Part model, mm, in its own coordinate system. Face numbers are marked on the shaded views. A direction names the side the tool comes from. Give positions to 0.01 mm unless a question says otherwise; leave off trailing zeros. Order: outer loops, then holes, each group sorted by start corner. A loop starts at its lowest first (then second) coordinate and runs counter-clockwise, first axis right, second up. Notation, with made-up numbers: M 21.5,75 L 56.5,75 A16 cw 56.5,80 Z; hole C 38,31.25 d4. An arc over 180 degrees is marked long. Return JSON: item names as keys, results as strings.
from build123d import *

# Parameters (mm, degrees)
SKETCH1_R     = 6.55
BODY_DEPTH    = 7.3
FLOOR_2_DEPTH = 2.2


with BuildPart() as part:
    # Sketch1 → Body (new body)
    with BuildSketch(Plane(origin=(0, 0, 0), x_dir=(1, 0, 0), z_dir=(0, 1, 0))):
        with BuildLine():
            Line((3, -8.006403687), (15.495614035, -3.324296268))
            ThreePointArc((15.495614035, -3.324296268), (17.8, 0), (15.495614035, 3.324296268))
            Line((15.495614035, 3.324296268), (3, 8.006403687))
            ThreePointArc((3, 8.006403687), (-0.436058681, 8.538873042), (-3.8, 7.659144861))
            Line((-3.8, 7.659144861), (-8.7, 5.228064063))
            Line((-8.7, 5.228064063), (-8.7, -5.228064063))
            Line((-8.7, -5.228064063), (-3.8, -7.659144861))
            ThreePointArc((-3.8, -7.659144861), (-0.436058681, -8.538873042), (3, -8.006403687))
        make_face()
        with Locations(Location((0, 0, 0), (0, 0, 270))):
            Circle(SKETCH1_R, mode=Mode.SUBTRACT)
        with BuildLine():
            Line((11.25, 1.55), (14.25, 1.55))
            ThreePointArc((14.25, 1.55), (15.8, 0), (14.25, -1.55))
            Line((14.25, -1.55), (11.25, -1.55))
            ThreePointArc((11.25, -1.55), (9.7, 0), (11.25, 1.55))
        make_face(mode=Mode.SUBTRACT)
    extrude(amount=BODY_DEPTH)

    # Sketch1<4> → Floor 2 (add)
    with BuildSketch(Plane(origin=(0, 0, 0), x_dir=(1, 0, 0), z_dir=(0, 1, 0))):
        with BuildLine():
            ThreePointArc((6.55, 0), (6.413226158, 1.33155182), (6.008616718, 2.607494034))
            Line((6.008616718, 2.607494034), (1.596491228, 4.260717752))
            ThreePointArc((1.596491228, 4.260717752), (3.73942075, 2.592148232), (4.55, 0))
            ThreePointArc((4.55, 0), (2.398060559, -3.866756464), (-2.022222222, -4.075919195))
            Line((-2.022222222, -4.075919195), (-6.242982203, -1.981835819))
            ThreePointArc((-6.242982203, -1.981835819), (-4.972324895, -4.263623476), (-2.911111111, -5.867532028))
            ThreePointArc((-2.911111111, -5.867532028), (-0.33405665, -6.541475839), (2.298245614, -6.133560719))
            ThreePointArc((2.298245614, -6.133560719), (5.383122178, -3.731554048), (6.55, 0))
        make_face()
        with BuildLine():
            Line((1.596491228, 4.260717752), (6.008616718, 2.607494034))
            ThreePointArc((6.008616718, 2.607494034), (4.512125554, 4.747970407), (2.298245614, 6.133560719))
            ThreePointArc((2.298245614, 6.133560719), (-0.33405665, 6.541475839), (-2.911111111, 5.867532028))
            ThreePointArc((-2.911111111, 5.867532028), (-6.029303442, 2.559296778), (-6.242982203, -1.981835819))
            Line((-6.242982203, -1.981835819), (-2.022222222, -4.075919195))
            ThreePointArc((-2.022222222, -4.075919195), (-4.173750186, 1.811714488), (1.596491228, 4.260717752))
        make_face()
    extrude(amount=FLOOR_2_DEPTH)


solid = part.part
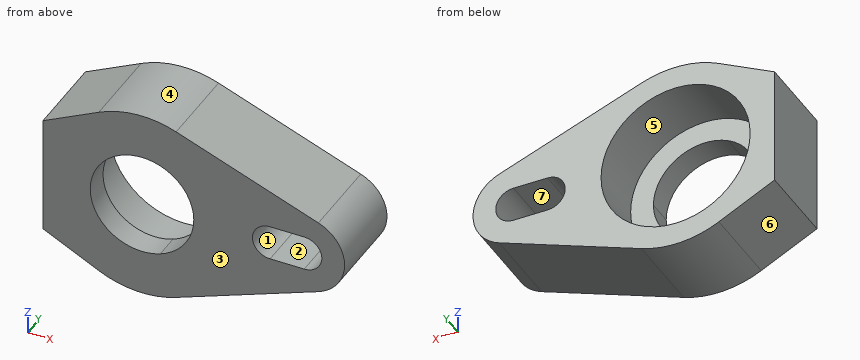
Q1. Band-saw the part on D-D (y = 5.5). Give the cut face in (x, z).
Established:
{"outline": "M -8.7,-5.23 L -3.8,-7.66 A8.55 ccw 3,-8.01 L 15.5,-3.32 A3.55 ccw 15.5,3.32 L 3,8.01 A8.55 ccw -3.8,7.66 L -8.7,5.23 Z; hole C 0,0 d13.1; hole M 11.25,-1.55 L 14.25,-1.55 A1.55 ccw 14.25,1.55 L 11.25,1.55 A1.55 ccw Z"}
Q2. Pin check, flat tips, straight feed: pin 1 (1.5 mm diameter, centred on x = -3.5, z = -2, fed in from -Y); pin 2 (3.5 mm diameter, centred on x = 13.5, y = 5.5, fed in from -Z); pin 3 (1.5 mm diameter, centred on x = 12.5, y = 2, fed in from +Z). Stop position of each tip, or through.
Established:
{"pin 1": "stops at y = 0", "pin 2": "stops at z = -4.73", "pin 3": "stops at z = 4.73"}
Q3. Band-saw the part on B-B (z = 1). Give the cut face in (x, y).
Established:
{"outline": "M -8.7,0 L -4.44,0 L -4.44,2.2 L -6.47,2.2 L -6.47,7.3 L -8.7,7.3 Z; M 4.44,0 L 10.07,0 L 10.07,7.3 L 6.47,7.3 L 6.47,2.2 L 4.44,2.2 Z; M 15.43,0 L 17.66,0 L 17.66,7.3 L 15.43,7.3 Z"}
Q4. Probe line 1 along X through (y, z) = (4, 0); line 2 along Z through (x, y) = (0, 3.8); line 3 along Y through (x, z) = (1, 4.5). List the from-to ranges inside material, lowest first.
Established:
{"line 1": "x = -8.7 to -6.55, 6.55 to 9.7, 15.8 to 17.8", "line 2": "z = -8.55 to -6.55, 6.55 to 8.55", "line 3": "y = 0 to 2.2"}
Q5. Band-saw the part on A-A (y = 1.25). Give the cut face in (x, z), then the cut area to 3 significant figures.
Established:
{"outline": "M -8.7,-5.23 L -3.8,-7.66 A8.55 ccw 3,-8.01 L 15.5,-3.32 A3.55 ccw 15.5,3.32 L 3,8.01 A8.55 ccw -3.8,7.66 L -8.7,5.23 Z; hole C 0,0 d9.1; hole M 11.25,-1.55 L 14.25,-1.55 A1.55 ccw 14.25,1.55 L 11.25,1.55 A1.55 ccw Z", "area": "247 mm²"}
Q6. 3-axis set-ups, long thin cutter, end or side, ignore diameter. For the marked faces 5, 6 and 7: which of +Z, -Z, +X, -X, +Y, -Y reach the whole face in a straight line?
Established:
{"face 5": "+Y", "face 6": "-Z, -X, +Y, -Y", "face 7": "+Y, -Y"}
Q7. Band-saw the part on C-C (x = 10.5). Give the cut face in (y, z).
Established:
{"outline": "M 0,-5.2 L 7.3,-5.2 L 7.3,-1.36 L 0,-1.36 Z; M 0,1.36 L 7.3,1.36 L 7.3,5.2 L 0,5.2 Z"}
Q8. Two-plate mould, pull along Z, no slides. Class the marked faces 1, 2, 3 and 4: +Z half, -Z half, draft (parallel to the pull), parting line (faces both ways), or undercut.
Established:
{"face 1": "undercut", "face 2": "undercut", "face 3": "draft", "face 4": "+Z half"}
